The figure shows three views and two pictorial views of one solid part (mm, origin at its lowest corner). Answer the questions. Coordinates: 2 decimals unless noted, no trailing zeros. Loops run counter-clockwise (first coordinate to the right, second up) from the corner with the lowest first, then second, coordinate; pieces in that order, holes last.
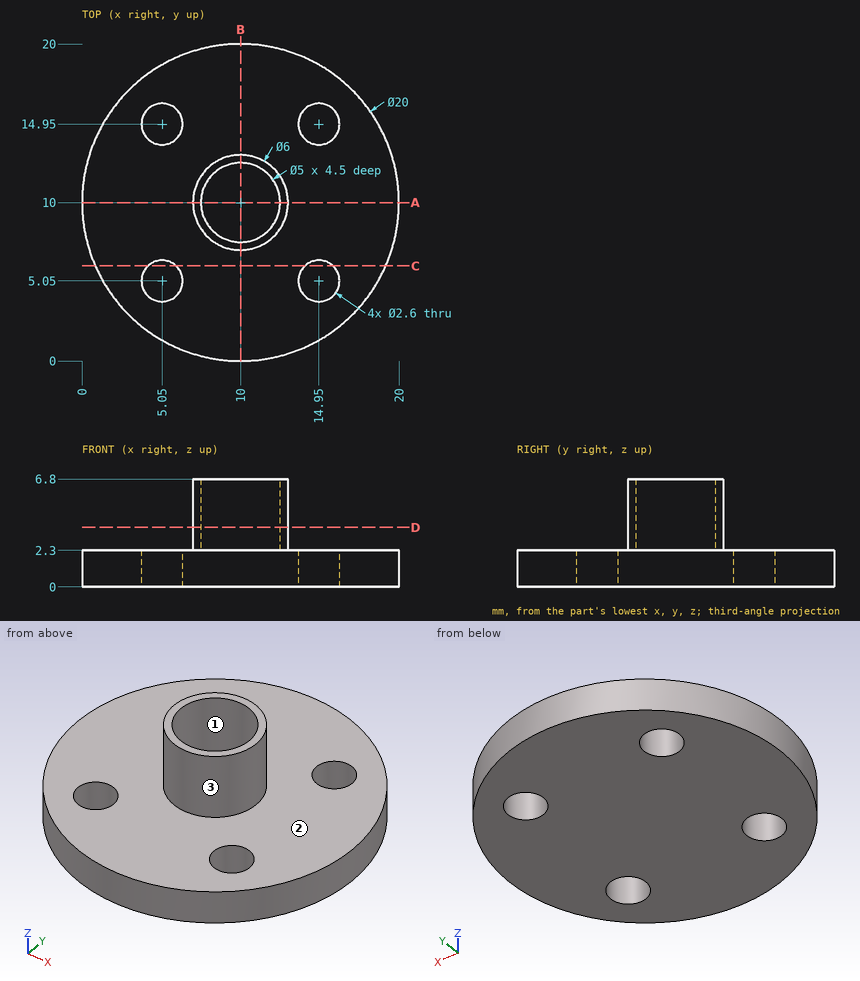
Q1. Flat-ended cylindrical pins translate along their axes: pin 1 Ø4.5 at (x, y) = (10, 10) entering from +Z; pin 2 Ø3 at (x, z) = (13.5, 5) entering from +Y (1 decimal); pin 3 Ø3 at (x, z) = (14, 1.5) entering from +Y. Find the tip coordinate at first contact, or state that the pin passes through.
Findings below:
pin 1: stops at z = 2.3
pin 2: stops at y = 12.2
pin 3: stops at y = 19.68
Q2. Straight lines are drawn through the part: probe 1 along X at (y, z) = (14, 0.75) (1 decimal); probe 2 along Z at (x, y) = (8, 17.25); probe 3 along X at (y, z) = (5.25, 1.25) (1 decimal). For each, find the intervals that lie inside material, in ascending order.
Findings below:
probe 1: x = 0.8 to 4.2, 5.9 to 14.1, 15.8 to 19.2
probe 2: z = 0 to 2.3
probe 3: x = 1.2 to 3.8, 6.3 to 13.7, 16.2 to 18.8
Q3. A cutting plane is placed at A-A (y = 10). Give the vertices of the cut face in (x, z), then the cut area to 3 significant figures.
Findings below:
outline: (0, 0) - (20, 0) - (20, 2.3) - (13, 2.3) - (13, 6.8) - (12.5, 6.8) - (12.5, 2.3) - (7.5, 2.3) - (7.5, 6.8) - (7, 6.8) - (7, 2.3) - (0, 2.3) - close
area: 50.5 mm2
Q4. A cutting plane is placed at D-D (z = 3.75). Give the vertices of the cut face in (x, y).
Findings below:
outline: circle Ø6 at (10, 10); hole circle Ø5 at (10, 10)
Q5. A cutting plane is placed at C-C (y = 6). Give the vertices of the cut face in (x, z) (1 decimal).
Findings below:
outline: (0.8, 0) - (4.2, 0) - (4.2, 2.3) - (0.8, 2.3) - close; (5.9, 0) - (14.1, 0) - (14.1, 2.3) - (5.9, 2.3) - close; (15.8, 0) - (19.2, 0) - (19.2, 2.3) - (15.8, 2.3) - close
Q6. Determine the mould class of the marked faces 1, 2 and 3 for opening direction X: +X half, -X half, draft (parallel to the pull), parting line (faces both ways), or undercut.
Findings below:
face 1: undercut
face 2: draft
face 3: parting line
